```python
from build123d import *

# Parameters (mm, degrees)
F0_W     = 53.1802996993
F0_H     = 46.4934445918
F0_R     = 2.5936293998
F1_DEPTH = 25.4
F2_W     = 46.8302996993
F2_H     = 40.1434445918
F2_R     = 2.5936293998
F3_DEPTH = 12.7
F4_W     = 31.6434130073
F4_H     = 47.7159637958
F4_W_2   = 96.1484760046
F5_DEPTH = 5.08
F4_W_3   = 7.8468769789
F4_H_2   = 9.7482251003


with BuildPart() as f1:
    # F0 (on Front) → F1 (new body)
    with BuildSketch(Plane.XZ):
        with Locations((6.9469735026, 14.2225120217)):
            Rectangle(F0_W, F0_H)
        with Locations((0, 14.2225120217)):
            Circle(F0_R, mode=Mode.SUBTRACT)
    extrude(amount=F1_DEPTH)

    # F2 (on face) → F3 (join)
    with BuildSketch(Plane.XZ.offset(25.4)):
        with Locations((3.7719735026, 17.3975120217)):
            Rectangle(F2_W, F2_H)
        with Locations((0, 14.2225120217)):
            Circle(F2_R, mode=Mode.SUBTRACT)
    extrude(amount=F3_DEPTH)

    # F4 (on Front) → F5 (join)
    with BuildSketch(Plane.XZ):
        with Locations((85.3468738496, 19.3866211921)):
            Rectangle(F4_W, F4_H)
        Polygon((69.525167346, -45.0122542679), (69.525167346, -4.4713607058), (-26.6233086586, -4.4713607058), (-26.6233086586, 43.24460309), (69.525167346, 43.24460309), (69.525167346, 73.4572783113), (-55.6312203407, 73.4572783113), (-55.6312203407, -45.0122542679), align=None)
        with Locations((21.4509293437, 19.3866211921)):
            Rectangle(F4_W_2, F4_H)
    extrude(amount=-F5_DEPTH)


with BuildPart() as f5:
    # F4 (on Front) → F5, piece 2 (new body)
    with BuildSketch(Plane.XZ):
        with Locations((111.8179112673, 1.5299557708)):
            Rectangle(F4_W_3, F4_H_2)
    extrude(amount=-F5_DEPTH)


solid = f1.part
```
Source: CAD feature listing. Evaluate the final solid. Frame: model axes, mm. A direction names the side the tool comes from. Give positions to 0.01 mm unless a question says otherwise; leave off trailing zeros. Loops run counter-clockwise (first coordinate to the right, second up) from the corner with the lowest first, then second, coordinate; pieces in that order, holes last. Notation, with made-up numbers: (88.5, -30) - (94.5, -30) arc R17 ccw to (94.5, 3) - close; hole circle Ø4 at (60, 37.5). An arc over 180 degrees is marked (long way). Use CSV: the item, a comma, the result in double quotes.
1) Pin query (flat end, axial travel): P1, Ø19, axis at y = -24, z = 20, coming from the -X side; P2, Ø4, axis at y = 3.5, z = 62, coming from the +X side; P3, Ø6, axis at x = 5, z = -19, coming from the -Y side. Return the tip coordinate at first contact, or that it passes through.
Worked out:
P1,"stops at x = -19.64"
P2,"stops at x = 69.53"
P3,"stops at y = 0"
2) Cut plane A-A (x = 25). Output: boundary loops of the cut face in (y, z).
Worked out:
outline,"(-38.1, -2.67) - (-25.4, -2.67) - (-25.4, -9.02) - (0, -9.02) - (0, -45.01) - (5.08, -45.01) - (5.08, 73.46) - (0, 73.46) - (0, 37.47) - (-38.1, 37.47) - close"
3) Cut plane D-D (x = 0). Output: boundary loops of the cut face in (y, z).
Worked out:
outline,"(-38.1, -2.67) - (-25.4, -2.67) - (-25.4, -9.02) - (0, -9.02) - (0, -45.01) - (5.08, -45.01) - (5.08, 73.46) - (0, 73.46) - (0, 37.47) - (-38.1, 37.47) - (-38.1, 16.82) - (0, 16.82) - (0, 11.63) - (-38.1, 11.63) - close"
4) Set-up query: faces 1 (the flat face through (3, -32, -2.674)), 2 (the flat face through (85, 3, -4.471)), 3 (the flat face through (0, 0, 14)), 4 (the flat face through (27.187, -32, 17)). Return all of +Z, -Z, +X, -X, +Y, -Y with unobstructed straight access to the full face (end or side cutting, diameter ignored); none if empty.
Worked out:
face 1,"-Z, +X, -X, -Y"
face 2,"-Z, +X, +Y, -Y"
face 3,"-Y"
face 4,"+Z, -Z, +X, -Y"
5) Cut plane B-B (y = 2.5). Output: boundary loops of the cut face in (x, z).
Worked out:
outline,"(-55.63, -45.01) - (69.53, -45.01) - (69.53, -4.47) - (101.17, -4.47) - (101.17, 43.24) - (69.53, 43.24) - (69.53, 73.46) - (-55.63, 73.46) - close"
6) Mould query, pull axis X, two halves, no side actions, for faces 5 (the flat face through (-19.643, -19, 14)), 6 (the flat face through (3, -38.1, 18)), 7 (the cylindrical face through (-0.6, -18.8, 11.7)), 8 (the flat face through (33.537, -13, 14)). Classes: +X half, -X half, draft (parallel to the pull), parting line (faces both ways), or undercut.
Worked out:
face 5,"-X half"
face 6,"draft"
face 7,"undercut"
face 8,"+X half"
7) Cut plane C-C (z = 27). Output: boundary loops of the cut face in (x, y).
Worked out:
outline,"(-55.63, 0) - (-19.64, 0) - (-19.64, -38.1) - (27.19, -38.1) - (27.19, -25.4) - (33.54, -25.4) - (33.54, 0) - (101.17, 0) - (101.17, 5.08) - (-55.63, 5.08) - close"
8) Line query: line 1 (Z direction, x = 0, y = -29); line 2 (Z direction, x = 0, y = -14); line 3 (X direction, y = -22.5, z = 8). Output: solid intervals per line, ascending.
Worked out:
line 1,"z = -2.67 to 11.63, 16.82 to 37.47"
line 2,"z = -9.02 to 11.63, 16.82 to 37.47"
line 3,"x = -19.64 to 33.54"
